Read the model definition and answer for the solid it produces. Units are mm, in the model's axes. Face numbers are marked on the shaded views. A direction names the side the tool comes from. Coordinates: 2 decimals unless noted, no trailing zeros. Loops run counter-clockwise (first coordinate to the right, second up) from the corner with the lowest first, then second, coordinate; pieces in that order, holes last. Notation, with made-up numbers: M -1.75,76 L 37.25,76 A9 ccw 37.25,84 Z; hole C -33.5,-5 d5. An arc over 180 degrees is marked long. Use one line per item in the form item = value. Start each with the question number.
1. For a pull along X with two mould halves and no side action, classify the marked faces 4, 5, 6 and 7 as released by +X, released by -X, zero draft, split by the parting line, or undercut.
2. Find the intervals of material crossed by probe 1 along X at (y, z) = (27.15, 0); probe 2 along X at (y, z) = (1.7, 45); probe 3 along X at (y, z) = (45.5, 0), in increasing order. Write a range as [from, to].
3. Flat-ended cylindrical pins translate along their axes: pin 1 (4.5 mm diameter, centred on y = 28, z = -1.5, fed in from +X); pin 2 (1 mm diameter, centred on y = 33, z = -18, fed in from -X); pin 3 (8 mm diameter, centred on y = 13, z = -2.5, fed in from -X); pin 4 (2 mm diameter, centred on x = 20, y = 63.5, fed in from +Z). Find the tip coordinate at first contact, or state that the pin passes through.
4. The part is cut by section B-B (y = 46). Give the vertices of the cut face in (x, z).
5. The part is cut by section A-A (x = -55). Give the vertices of the cut face in (y, z).
6. The part is cut by section C-C (x = 0). Give the number of separate pieces and of enclosed holes in the cut face, plus the area to 3 significant figures.
7. A tool of negligible diameter and unlimited length cuts with its end or side. For the marked faces 1, 2 and 3, from which of +Z, -Z, +X, -X, +Y, -Y can it reach the whole face along a straight path? Write none if from no direction.
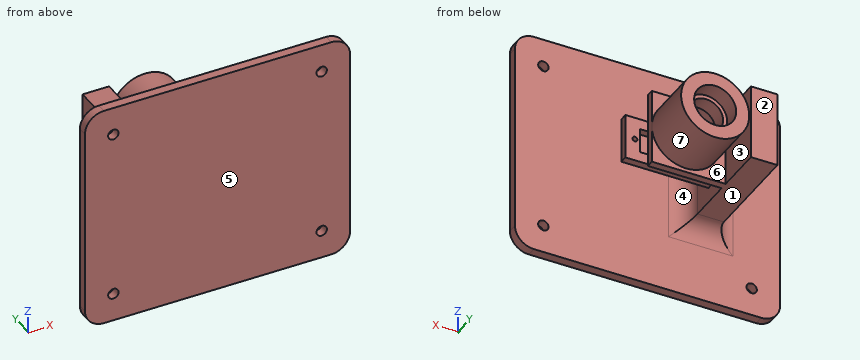
from build123d import *

# Parameters (mm, degrees)
BENCH_FOOTPRINT_140X120_DEPTH           = 5
BACKBONE_START                          = -20
BACKBONE_PROFILE_W                      = 14
BACKBONE_PROFILE_H                      = 63
BACKBONE_DEPTH                          = 40
SERVO_SHELF_START                       = 26
SERVO_SHELF_PROFILE_W                   = 60
SERVO_SHELF_PROFILE_H                   = 24
SERVO_SHELF_DEPTH                       = 4
SERVO_BODY_WINDOW_START                 = 25
SERVO_BODY_WINDOW_PROFILE_W             = 23.8
SERVO_BODY_WINDOW_PROFILE_H             = 13
SERVO_BODY_WINDOW_DEPTH                 = 90.560027933
YAW_SERVO_FASTENERS_START               = 25
YAW_SERVO_FASTENERS_PROFILE_R           = 1.3
YAW_SERVO_FASTENERS_DEPTH               = 90.560027933
BEARING_BRIDGE_START                    = 39
BEARING_BRIDGE_PROFILE_W                = 53
BEARING_BRIDGE_PROFILE_H                = 40
BEARING_BRIDGE_DEPTH                    = 4
BRIDGE_HORN_CLEARANCE_START             = 38
BRIDGE_HORN_CLEARANCE_PROFILE_R         = 14
BRIDGE_HORN_CLEARANCE_DEPTH             = 77.560027933
DRIVE_COLLAR_CHAMBER_START              = 43
DRIVE_COLLAR_CHAMBER_PROFILE_R          = 18
DRIVE_COLLAR_CHAMBER_PROFILE_R_2        = 14
DRIVE_COLLAR_CHAMBER_DEPTH              = 5
BEARING_TOWER_START                     = 48
BEARING_TOWER_PROFILE_R                 = 18
BEARING_TOWER_PROFILE_R_2               = 11.1
BEARING_TOWER_DEPTH                     = 24
BEARING_SEPARATION_SHOULDER_START       = 55
BEARING_SEPARATION_SHOULDER_PROFILE_R   = 11.1
BEARING_SEPARATION_SHOULDER_PROFILE_R_2 = 9
BEARING_SEPARATION_SHOULDER_DEPTH       = 8
BENCH_CLAMP_HOLES_START                 = -1
BENCH_CLAMP_HOLES_PROFILE_R             = 2.75
BENCH_CLAMP_HOLES_DEPTH                 = 118.978630527
FILLET1_R                               = 10


with BuildPart() as part:
    # Bench_footprint_140x120_profile → Bench_footprint_140x120 (new body)
    with BuildSketch(Plane(origin=(0, 0, 0), x_dir=(1, 0, 0), z_dir=(0, 1, 0))):
        with BuildLine():
            Line((-60, -60), (60, -60))
            ThreePointArc((60, -60), (67.071067812, -57.071067812), (70, -50))
            Line((70, -50), (70, 50))
            ThreePointArc((70, 50), (67.071067812, 57.071067812), (60, 60))
            Line((60, 60), (-60, 60))
            ThreePointArc((-60, 60), (-67.071067812, 57.071067812), (-70, 50))
            Line((-70, 50), (-70, -50))
            ThreePointArc((-70, -50), (-67.071067812, -57.071067812), (-60, -60))
        make_face()
    extrude(amount=BENCH_FOOTPRINT_140X120_DEPTH)

    # Backbone_profile → Backbone (add)
    with BuildSketch(Plane.XY.offset(BACKBONE_START)):
        with Locations((-28, 36.5)):
            Rectangle(BACKBONE_PROFILE_W, BACKBONE_PROFILE_H)
    extrude(amount=BACKBONE_DEPTH)

    # Servo_shelf_profile → Servo_shelf (add)
    with BuildSketch(Plane(origin=(0, 0, 0), x_dir=(1, 0, 0), z_dir=(0, 1, 0)).offset(SERVO_SHELF_START)):
        with Locations((-5, 0)):
            Rectangle(SERVO_SHELF_PROFILE_W, SERVO_SHELF_PROFILE_H)
    extrude(amount=SERVO_SHELF_DEPTH)

    # Servo_body_window_profile → Servo_body_window (cut, through all)
    with BuildSketch(Plane(origin=(0, 0, 0), x_dir=(1, 0, 0), z_dir=(0, 1, 0)).offset(SERVO_BODY_WINDOW_START)):
        with Locations((5.5, 0)):
            Rectangle(SERVO_BODY_WINDOW_PROFILE_W, SERVO_BODY_WINDOW_PROFILE_H)
    extrude(amount=SERVO_BODY_WINDOW_DEPTH, mode=Mode.SUBTRACT)

    # Yaw_servo_fasteners_profile → Yaw_servo_fasteners (cut, through all)
    with BuildSketch(Plane(origin=(0, 0, 0), x_dir=(1, 0, 0), z_dir=(0, 1, 0)).offset(YAW_SERVO_FASTENERS_START)):
        with Locations(Location((-9, 0, 0), (0, 0, 90))):
            Circle(YAW_SERVO_FASTENERS_PROFILE_R)
        with Locations(Location((20, 0, 0), (0, 0, 90))):
            Circle(YAW_SERVO_FASTENERS_PROFILE_R)
    extrude(amount=YAW_SERVO_FASTENERS_DEPTH, mode=Mode.SUBTRACT)

    # Bearing_bridge_profile → Bearing_bridge (add)
    with BuildSketch(Plane(origin=(0, 0, 0), x_dir=(1, 0, 0), z_dir=(0, 1, 0)).offset(BEARING_BRIDGE_START)):
        with Locations((-8.5, 0)):
            Rectangle(BEARING_BRIDGE_PROFILE_W, BEARING_BRIDGE_PROFILE_H)
    extrude(amount=BEARING_BRIDGE_DEPTH)

    # Bridge_horn_clearance_profile → Bridge_horn_clearance (cut, through all)
    with BuildSketch(Plane(origin=(0, 0, 0), x_dir=(1, 0, 0), z_dir=(0, 1, 0)).offset(BRIDGE_HORN_CLEARANCE_START)):
        with Locations(Location((0, 0, 0), (0, 0, 90))):
            Circle(BRIDGE_HORN_CLEARANCE_PROFILE_R)
    extrude(amount=BRIDGE_HORN_CLEARANCE_DEPTH, mode=Mode.SUBTRACT)

    # Drive_collar_chamber_profile → Drive_collar_chamber (add)
    with BuildSketch(Plane(origin=(0, 0, 0), x_dir=(1, 0, 0), z_dir=(0, 1, 0)).offset(DRIVE_COLLAR_CHAMBER_START)):
        Circle(DRIVE_COLLAR_CHAMBER_PROFILE_R)
        with Locations(Location((0, 0, 0), (0, 0, 90))):
            Circle(DRIVE_COLLAR_CHAMBER_PROFILE_R_2, mode=Mode.SUBTRACT)
    extrude(amount=DRIVE_COLLAR_CHAMBER_DEPTH)

    # Bearing_tower_profile → Bearing_tower (add)
    with BuildSketch(Plane(origin=(0, 0, 0), x_dir=(1, 0, 0), z_dir=(0, 1, 0)).offset(BEARING_TOWER_START)):
        Circle(BEARING_TOWER_PROFILE_R)
        with Locations(Location((0, 0, 0), (0, 0, 270))):
            Circle(BEARING_TOWER_PROFILE_R_2, mode=Mode.SUBTRACT)
    extrude(amount=BEARING_TOWER_DEPTH)

    # Bearing_separation_shoulder_profile → Bearing_separation_shoulder (add)
    with BuildSketch(Plane(origin=(0, 0, 0), x_dir=(1, 0, 0), z_dir=(0, 1, 0)).offset(BEARING_SEPARATION_SHOULDER_START)):
        with Locations(Location((0, 0, 0), (0, 0, 270))):
            Circle(BEARING_SEPARATION_SHOULDER_PROFILE_R)
        with Locations(Location((0, 0, 0), (0, 0, 270))):
            Circle(BEARING_SEPARATION_SHOULDER_PROFILE_R_2, mode=Mode.SUBTRACT)
    extrude(amount=BEARING_SEPARATION_SHOULDER_DEPTH)

    # Bench_clamp_holes_profile → Bench_clamp_holes (cut, through all)
    with BuildSketch(Plane(origin=(0, 0, 0), x_dir=(1, 0, 0), z_dir=(0, 1, 0)).offset(BENCH_CLAMP_HOLES_START)):
        with Locations(Location((-55, -45, 0), (0, 0, 90))):
            Circle(BENCH_CLAMP_HOLES_PROFILE_R)
        with Locations(Location((55, -45, 0), (0, 0, 90))):
            Circle(BENCH_CLAMP_HOLES_PROFILE_R)
        with Locations(Location((-55, 45, 0), (0, 0, 90))):
            Circle(BENCH_CLAMP_HOLES_PROFILE_R)
        with Locations(Location((55, 45, 0), (0, 0, 90))):
            Circle(BENCH_CLAMP_HOLES_PROFILE_R)
    extrude(amount=BENCH_CLAMP_HOLES_DEPTH, mode=Mode.SUBTRACT)

    # Fillet1
    fillet1_edges = [part.edges().sort_by_distance(p)[0] for p in [
        (-28, 5, -20),
        (-35, 5, 0),
        (-21, 5, 0),
        (-28, 5, 20),
    ]]
    fillet(fillet1_edges, radius=FILLET1_R)


solid = part.part
Computed values:
q1.face_4 = released by +X
q1.face_5 = zero draft
q1.face_6 = undercut
q1.face_7 = undercut
q2.probe_1 = [-35, -10.3], [-7.7, -6.4], [17.4, 18.7], [21.3, 25]
q2.probe_2 = [-70, -57.75], [-52.25, 52.25], [57.75, 70]
q2.probe_3 = [-35, -21], [-18, -14], [14, 18]
q3.pin_1 = 25
q3.pin_2 = -35
q3.pin_3 = -37
q3.pin_4 = through
q4.outline = M -35,-20 L -21,-20 L -21,20 L -35,20 Z; C 0,0 d36; hole C 0,0 d28
q5.outline = M 0,-60 L 5,-60 L 5,-47.75 L 0,-47.75 Z; M 0,-42.25 L 5,-42.25 L 5,42.25 L 0,42.25 Z; M 0,47.75 L 5,47.75 L 5,60 L 0,60 Z
q6.separate_pieces = 5
q6.enclosed_holes = 0
q6.area = 1,100 mm²
q7.face_1 = -Z, +X, -X, +Y
q7.face_2 = +Z, -Z, -X, +Y
q7.face_3 = +Z, -Z, +Y
